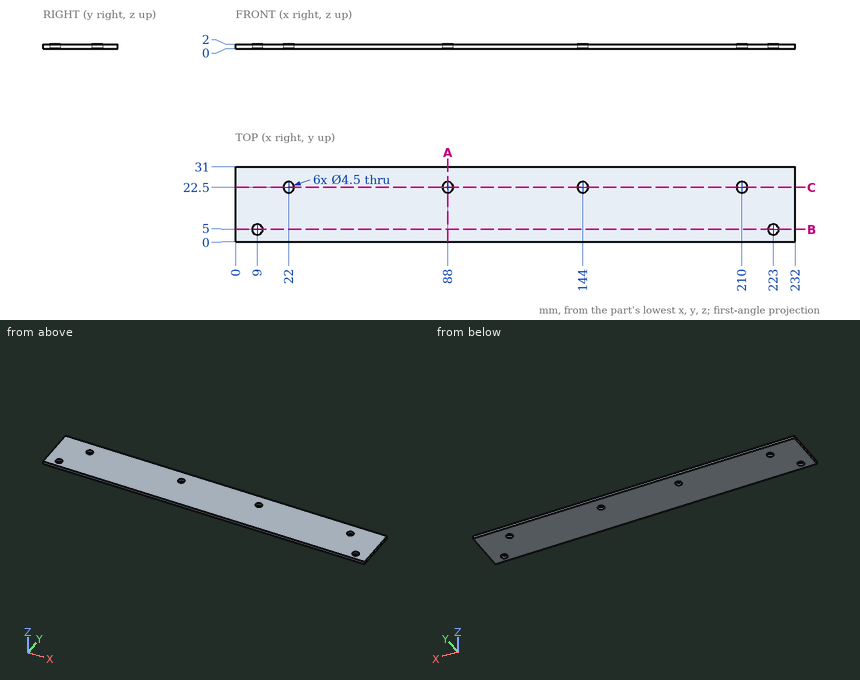
Here's the drawing with two shaded views (mm, measured from the low corner). I have some questions. Give positions to 0.01 mm unless a question says otherwise; leave off trailing zeros. Loops run counter-clockwise (first coordinate to the right, second up) from the corner with the lowest first, then second, coordinate; pieces in that order, holes last. Notation, with made-up numbers: (-17, -11.5) -> (-1, -11.5) arc R32 cw to (-1, 14.5) -> close; hole circle Ø11 at (78, -31.75). An arc over 180 degrees is marked (long way). Use one line per item in the form item = value.
1) If we section it at C-C (y = 22.5): Please give me the cut outline in (x, z).
Answers:
outline = (0, 0) -> (19.75, 0) -> (19.75, 2) -> (0, 2) -> close; (24.25, 0) -> (85.75, 0) -> (85.75, 2) -> (24.25, 2) -> close; (90.25, 0) -> (141.75, 0) -> (141.75, 2) -> (90.25, 2) -> close; (146.25, 0) -> (207.75, 0) -> (207.75, 2) -> (146.25, 2) -> close; (212.25, 0) -> (232, 0) -> (232, 2) -> (212.25, 2) -> close
2) If we section it at B-B (y = 5): Please give me the cut outline in (x, z).
Answers:
outline = (0, 0) -> (6.75, 0) -> (6.75, 2) -> (0, 2) -> close; (11.25, 0) -> (220.75, 0) -> (220.75, 2) -> (11.25, 2) -> close; (225.25, 0) -> (232, 0) -> (232, 2) -> (225.25, 2) -> close
3) Will these pins go through, and if not, where does the flat tip stop? pin 1 (2.5 mm diameter, centred on x = 22, y = 22.5, fed in from +Z); pin 2 (5 mm diameter, centred on x = 9, y = 5, fed in from -Z).
Answers:
pin_1 = through
pin_2 = 0
4) I need wall thicknesses on line 1 along Y through (x, z) = (88, 1.65); line 2 along X through (y, z) = (23, 0.5); line 3 along X through (y, z) = (4, 1.2). Which ranges of each line are inside material? Lowest first, please.
Answers:
line_1 = 0 to 20.25, 24.75 to 31
line_2 = 0 to 19.81, 24.19 to 85.81, 90.19 to 141.81, 146.19 to 207.81, 212.19 to 232
line_3 = 0 to 6.98, 11.02 to 220.98, 225.02 to 232
5) If we section it at A-A (x = 88): Please give me the cut outline in (y, z).
Answers:
outline = (0, 0) -> (20.25, 0) -> (20.25, 2) -> (0, 2) -> close; (24.75, 0) -> (31, 0) -> (31, 2) -> (24.75, 2) -> close
